Part model, mm, in its own coordinate system. A direction names the side the tool comes from. Round coordinates to 2 decimals unless told otherwise and drop trailing zeros. Loops run counter-clockwise (first coordinate to the right, second up) from the corner with the lowest first, then second, coordinate; pieces in that order, holes last.
(1) Cut at B-B on z = 4. List the corners of the cut face in (x, y).
(2) Flat gauge pins, fed straight in: pin 1 (0.6 mm diameter, centred on y = 3.5, z = 93.5, fed in from -X); pin 2 (4 mm diameter, centred on x = -48.25, z = -39.44, fed in from +Y); pin 3 (2 mm diameter, centred on y = 3.5, z = -42.5, fed in from -X); pin 4 (3 mm diameter, centred on x = 126, y = 3.5, fed in from +Z). Where does each tip first touch, or does it go through?
(3) Probe probe 1 along X at (y, z) = (0.45, 50); probe 2 along X at (y, z) = (0.65, 21); probe 3 along X at (y, z) = (5.25, 11.5). List the from-to ranges inside material, lowest first.
(4) Cut at C-C on y = 4.3. Count the separate pieces of the cut face and the enclosed holes in it, then the cut area to 3 significant figures.
(5) Cut at D-D on z = 47.5. List the corners of the cut face in (x, y), then the cut area to 3 significant figures.
(6) Tool access for faces 4 (the face through (-94, 3, 79.635)), 5 (the face through (-59.509, 3, 26)), 6 (the face through (-95, 3, -28.523)): list every direction of +Z, -Z, +X, -X, +Y, -Y with a clear straight run to the whole face (end or side of a thin tool).
(7) Cut at A-A on x = 2. List the corners of the cut face in (y, z), then the cut area to 3 significant figures.
(8) Mould opens along X. For faces 1 (the face through (93.001, 3, 26)), 2 (the face through (144.454, 2.833, -26.35)), 3 (the face through (14, 0, 64)) say: +X half, -X half, draft (parallel to the pull), parting line (faces both ways), or undercut.
from build123d import *

# Parameters (mm, degrees)
BOSS_EXTRUDE1_DEPTH = 5.588
SKETCH2_R           = 2.159
CUT_EXTRUDE1_DEPTH  = 158.413946399
SKETCH3_W           = 152.51
SKETCH3_H           = 61.34
CUT_EXTRUDE2_DEPTH  = 158.413946399
BOSS_EXTRUDE2_DEPTH = 5.588
BOSS_EXTRUDE3_DEPTH = 5.588
SKETCH7_R           = 1.75
CUT_EXTRUDE4_DEPTH  = 187.865769606
SKETCH8_R           = 1.75
CUT_EXTRUDE6_DEPTH  = 187.865769606
SKETCH9_R           = 1.75
CUT_EXTRUDE8_DEPTH  = 187.865769606
CUT_EXTRUDE9_DEPTH  = 187.865769606
FILLET1_R           = 3


with BuildPart() as part:
    # Sketch1 → Boss-Extrude1 (new body)
    with BuildSketch(Plane(origin=(0, 0, 0), x_dir=(1, 0, 0), z_dir=(0, 1, 0))):
        Polygon((-73.254183378, 28.522688753), (-37.333158894, 64.443713237), (70.824792138, 64.443713237), (106.745816622, 28.522688753), (106.745816622, -79.635262279), (70.824792138, -115.556286763), (-37.333158894, -115.556286763), (-73.254183378, -79.635262279), align=None)
    extrude(amount=BOSS_EXTRUDE1_DEPTH)

    # Sketch2 → Cut-Extrude1 (cut, through all)
    with BuildSketch(Plane(origin=(0, 5.588, 0), x_dir=(1, 0, 0), z_dir=(0, 1, 0))):
        with Locations(Location((-48.254183378, 39.443713237, 0), (0, 0, 270))):
            Circle(SKETCH2_R)
        with Locations(Location((-30.576513848, 21.766043708, 0), (0, 0, 270))):
            Circle(SKETCH2_R)
        with Locations(Location((-48.254183378, -90.556286763, 0), (0, 0, 270))):
            Circle(SKETCH2_R)
        with Locations(Location((-30.576513848, -72.878617233, 0), (0, 0, 270))):
            Circle(SKETCH2_R)
        with Locations(Location((64.068147093, 21.766043708, 0), (0, 0, 270))):
            Circle(SKETCH2_R)
        with Locations(Location((81.745816622, 39.443713237, 0), (0, 0, 270))):
            Circle(SKETCH2_R)
        with Locations(Location((64.068147093, -72.878617233, 0), (0, 0, 270))):
            Circle(SKETCH2_R)
        with Locations(Location((81.745816622, -90.556286763, 0), (0, 0, 270))):
            Circle(SKETCH2_R)
    extrude(amount=-CUT_EXTRUDE1_DEPTH, mode=Mode.SUBTRACT)

    # Sketch3 → Cut-Extrude2 (cut, through all)
    with BuildSketch(Plane(origin=(0, 5.588, 0), x_dir=(1, 0, 0), z_dir=(0, 1, 0))):
        with Locations((16.745816622, -25.556286763)):
            Rectangle(SKETCH3_W, SKETCH3_H)
    extrude(amount=-CUT_EXTRUDE2_DEPTH, mode=Mode.SUBTRACT)

    # Sketch5 → Boss-Extrude2 (add)
    with BuildSketch(Plane(origin=(0, 5.588, 0), x_dir=(1, 0, 0), z_dir=(0, 1, 0))):
        with BuildLine():
            Line((-73.254183378, -79.635262279), (-115.634183378, -79.635262279))
            ThreePointArc((-115.634183378, -79.635262279), (-121.02233705, -77.403415951), (-123.254183378, -72.015262279))
            Line((-123.254183378, -72.015262279), (-123.254183378, 20.902688753))
            ThreePointArc((-123.254183378, 20.902688753), (-121.02233705, 26.290842426), (-115.634183378, 28.522688753))
            Line((-115.634183378, 28.522688753), (-73.254183378, 28.522688753))
            Line((-73.254183378, 28.522688753), (-73.254183378, -79.635262279))
        make_face()
    extrude(amount=-BOSS_EXTRUDE2_DEPTH)

    # Sketch6 → Boss-Extrude3 (add)
    with BuildSketch(Plane(origin=(0, 5.588, 0), x_dir=(1, 0, 0), z_dir=(0, 1, 0))):
        with BuildLine():
            Line((106.745816622, 28.522688753), (139.125816622, 28.522688753))
            ThreePointArc((139.125816622, 28.522688753), (144.513970295, 26.290842426), (146.745816622, 20.902688753))
            Line((146.745816622, 20.902688753), (146.745816622, -72.015262279))
            ThreePointArc((146.745816622, -72.015262279), (144.513970295, -77.403415951), (139.125816622, -79.635262279))
            Line((139.125816622, -79.635262279), (106.745816622, -79.635262279))
            Line((106.745816622, -79.635262279), (106.745816622, 28.522688753))
        make_face()
    extrude(amount=-BOSS_EXTRUDE3_DEPTH)

    # Sketch7 → Cut-Extrude4 (cut, through all)
    with BuildSketch(Plane(origin=(0, 5.588, 0), x_dir=(1, 0, 0), z_dir=(0, 1, 0))):
        with Locations(Location((110.045816622, -10.356286763, 0), (0, 0, 270))):
            Circle(SKETCH7_R)
        with Locations(Location((134.045816622, -10.356286763, 0), (0, 0, 270))):
            Circle(SKETCH7_R)
        with Locations(Location((110.045816622, -40.756286763, 0), (0, 0, 270))):
            Circle(SKETCH7_R)
        with Locations(Location((134.045816622, -40.756286763, 0), (0, 0, 270))):
            Circle(SKETCH7_R)
    extrude(amount=-CUT_EXTRUDE4_DEPTH, mode=Mode.SUBTRACT)

    # Sketch8 → Cut-Extrude6 (cut, through all)
    with BuildSketch(Plane(origin=(0, 5.588, 0), x_dir=(1, 0, 0), z_dir=(0, 1, 0))):
        with Locations(Location((-108.854183378, -25.556286763, 0), (0, 0, 270))):
            Circle(SKETCH8_R)
        with Locations(Location((-86.854183378, -25.556286763, 0), (0, 0, 270))):
            Circle(SKETCH8_R)
        with BuildLine():
            Line((-106.154183378, -24.006705166), (-106.154183378, -27.10586836))
            ThreePointArc((-106.154183378, -27.10586836), (-97.854183378, -53.606286763), (-89.554183378, -27.10586836))
            Line((-89.554183378, -27.10586836), (-89.554183378, -24.006705166))
            ThreePointArc((-89.554183378, -24.006705166), (-97.854183378, 2.493713237), (-106.154183378, -24.006705166))
        make_face()
    extrude(amount=-CUT_EXTRUDE6_DEPTH, mode=Mode.SUBTRACT)

    # Sketch9 → Cut-Extrude8 (cut, through all)
    with BuildSketch(Plane(origin=(0, 5.588, 0), x_dir=(1, 0, 0), z_dir=(0, 1, 0))):
        with Locations(Location((-53.254183378, 13.923713237, 0), (0, 0, 270))):
            Circle(SKETCH9_R)
        with Locations(Location((-43.254183378, 13.923713237, 0), (0, 0, 270))):
            Circle(SKETCH9_R)
        with Locations(Location((-33.254183378, 13.923713237, 0), (0, 0, 270))):
            Circle(SKETCH9_R)
        with Locations(Location((-23.254183378, 13.923713237, 0), (0, 0, 270))):
            Circle(SKETCH9_R)
        with Locations(Location((-13.254183378, 13.923713237, 0), (0, 0, 270))):
            Circle(SKETCH9_R)
        with Locations(Location((-3.254183378, 13.923713237, 0), (0, 0, 270))):
            Circle(SKETCH9_R)
        with Locations(Location((6.745816622, 13.923713237, 0), (0, 0, 270))):
            Circle(SKETCH9_R)
        with Locations(Location((16.745816622, 13.923713237, 0), (0, 0, 270))):
            Circle(SKETCH9_R)
        with Locations(Location((26.745816622, 13.923713237, 0), (0, 0, 270))):
            Circle(SKETCH9_R)
        with Locations(Location((36.745816622, 13.923713237, 0), (0, 0, 270))):
            Circle(SKETCH9_R)
        with Locations(Location((46.745816622, 13.923713237, 0), (0, 0, 270))):
            Circle(SKETCH9_R)
        with Locations(Location((56.745816622, 13.923713237, 0), (0, 0, 270))):
            Circle(SKETCH9_R)
        with Locations(Location((66.745816622, 13.923713237, 0), (0, 0, 270))):
            Circle(SKETCH9_R)
        with Locations(Location((76.745816622, 13.923713237, 0), (0, 0, 270))):
            Circle(SKETCH9_R)
        with Locations(Location((86.745816622, 13.923713237, 0), (0, 0, 270))):
            Circle(SKETCH9_R)
        with Locations(Location((-53.254183378, -65.036286763, 0), (0, 0, 270))):
            Circle(SKETCH9_R)
        with Locations(Location((-43.254183378, -65.036286763, 0), (0, 0, 270))):
            Circle(SKETCH9_R)
        with Locations(Location((-33.254183378, -65.036286763, 0), (0, 0, 270))):
            Circle(SKETCH9_R)
        with Locations(Location((-23.254183378, -65.036286763, 0), (0, 0, 270))):
            Circle(SKETCH9_R)
        with Locations(Location((-13.254183378, -65.036286763, 0), (0, 0, 270))):
            Circle(SKETCH9_R)
        with Locations(Location((-3.254183378, -65.036286763, 0), (0, 0, 270))):
            Circle(SKETCH9_R)
        with Locations(Location((6.745816622, -65.036286763, 0), (0, 0, 270))):
            Circle(SKETCH9_R)
        with Locations(Location((16.745816622, -65.036286763, 0), (0, 0, 270))):
            Circle(SKETCH9_R)
        with Locations(Location((26.745816622, -65.036286763, 0), (0, 0, 270))):
            Circle(SKETCH9_R)
        with Locations(Location((36.745816622, -65.036286763, 0), (0, 0, 270))):
            Circle(SKETCH9_R)
        with Locations(Location((46.745816622, -65.036286763, 0), (0, 0, 270))):
            Circle(SKETCH9_R)
        with Locations(Location((56.745816622, -65.036286763, 0), (0, 0, 270))):
            Circle(SKETCH9_R)
        with Locations(Location((66.745816622, -65.036286763, 0), (0, 0, 270))):
            Circle(SKETCH9_R)
        with Locations(Location((76.745816622, -65.036286763, 0), (0, 0, 270))):
            Circle(SKETCH9_R)
        with Locations(Location((86.745816622, -65.036286763, 0), (0, 0, 270))):
            Circle(SKETCH9_R)
    extrude(amount=-CUT_EXTRUDE8_DEPTH, mode=Mode.SUBTRACT)

    # Sketch10 → Cut-Extrude9 (cut, through all)
    with BuildSketch(Plane(origin=(0, 5.588, 0), x_dir=(1, 0, 0), z_dir=(0, 1, 0))):
        with BuildLine():
            Line((11.245816622, 45.443713237), (22.245816622, 45.443713237))
            ThreePointArc((22.245816622, 45.443713237), (23.660030185, 44.8579268), (24.245816622, 43.443713237))
            Line((24.245816622, 43.443713237), (24.245816622, 41.443713237))
            ThreePointArc((24.245816622, 41.443713237), (23.660030185, 40.029499675), (22.245816622, 39.443713237))
            Line((22.245816622, 39.443713237), (11.245816622, 39.443713237))
            ThreePointArc((11.245816622, 39.443713237), (9.83160306, 40.029499675), (9.245816622, 41.443713237))
            Line((9.245816622, 41.443713237), (9.245816622, 43.443713237))
            ThreePointArc((9.245816622, 43.443713237), (9.83160306, 44.8579268), (11.245816622, 45.443713237))
        make_face()
        with BuildLine():
            Line((11.245816622, -90.556286763), (22.245816622, -90.556286763))
            ThreePointArc((22.245816622, -90.556286763), (23.660030185, -91.1420732), (24.245816622, -92.556286763))
            Line((24.245816622, -92.556286763), (24.245816622, -94.556286763))
            ThreePointArc((24.245816622, -94.556286763), (23.660030185, -95.970500325), (22.245816622, -96.556286763))
            Line((22.245816622, -96.556286763), (11.245816622, -96.556286763))
            ThreePointArc((11.245816622, -96.556286763), (9.83160306, -95.970500325), (9.245816622, -94.556286763))
            Line((9.245816622, -94.556286763), (9.245816622, -92.556286763))
            ThreePointArc((9.245816622, -92.556286763), (9.83160306, -91.1420732), (11.245816622, -90.556286763))
        make_face()
    extrude(amount=-CUT_EXTRUDE9_DEPTH, mode=Mode.SUBTRACT)

    # Fillet1
    fillet1_edges = [part.edges().sort_by_distance(p)[0] for p in [
        (-59.509183378, 2.794, 56.226286763),
        (-59.509183378, 2.794, -5.113713237),
        (93.000816622, 2.794, -5.113713237),
        (93.000816622, 2.794, 56.226286763),
    ]]
    fillet(fillet1_edges, radius=FILLET1_R)


solid = part.part
Final values:
1. outline: (-123.25, 0) - (-109.97, 0) - (-109.97, 5.59) - (-123.25, 5.59) - close; (-85.74, 0) - (-59.51, 0) - (-59.51, 5.59) - (-85.74, 5.59) - close; (93, 0) - (146.75, 0) - (146.75, 5.59) - (93, 5.59) - close
2. pin 1: stops at x = -59.69
2. pin 2: passes through
2. pin 3: stops at x = -60.28
2. pin 4: stops at z = 79.64
3. probe 1: x = -123.25 to -107.44, -88.27 to -59.51, 93 to 146.75
3. probe 2: x = -123.25 to -109.33, -86.38 to -59.51, 93 to 146.75
3. probe 3: x = -123.25 to -112.39, -83.31 to -59.51, 93 to 108.72, 111.37 to 132.72, 135.37 to 146.75
4. separate pieces: 1
4. enclosed holes: 48
4. area: 28,200 mm2
5. outline: (-123.25, 0) - (-109.7, 0) - (-109.7, 5.59) - (-123.25, 5.59) - close; (-86, 0) - (-59.51, 0) - (-59.51, 5.59) - (-86, 5.59) - close; (93, 0) - (146.75, 0) - (146.75, 5.59) - (93, 5.59) - close
5. area: 524 mm2
6. face 4: +Z, -X, +Y, -Y
6. face 5: +Y, -Y
6. face 6: -Z, -X, +Y, -Y
7. outline: (0, -64.44) - (5.59, -64.44) - (5.59, -5.11) - (0, -5.11) - close; (0, 56.23) - (5.59, 56.23) - (5.59, 115.56) - (0, 115.56) - close
7. area: 663 mm2
8. face 1: undercut
8. face 2: +X half
8. face 3: draft
